from build123d import *

# Parameters (mm, degrees)
SKETCH1_W           = 39
SKETCH1_H           = 35
SKETCH1_R           = 1.912731322
BOSS_EXTRUDE1_DEPTH = 5
SKETCH2_R           = 2
BOSS_EXTRUDE2_DEPTH = 20
FILLET1_R           = 8


with BuildPart() as part:
    # Sketch1 → Boss-Extrude1 (new body)
    with BuildSketch(Plane.XY):
        Rectangle(SKETCH1_W, SKETCH1_H)
        with Locations((14.5, -12.5)):
            Circle(SKETCH1_R, mode=Mode.SUBTRACT)
        with Locations((14.5, 12.5)):
            Circle(SKETCH1_R, mode=Mode.SUBTRACT)
        with Locations((-14.5, -12.5)):
            Circle(SKETCH1_R, mode=Mode.SUBTRACT)
        with Locations((-14.5, 12.5)):
            Circle(SKETCH1_R, mode=Mode.SUBTRACT)
    extrude(amount=BOSS_EXTRUDE1_DEPTH)

    # Sketch2 → Boss-Extrude2 (add)
    with BuildSketch(Plane.XY.offset(5)):
        Circle(SKETCH2_R)
    extrude(amount=BOSS_EXTRUDE2_DEPTH)

    # Fillet1
    fillet1_edges = [part.edges().sort_by_distance(p)[0] for p in [
        (-2, 0, 5),
    ]]
    fillet(fillet1_edges, radius=FILLET1_R)


solid = part.part
Input: part model. Units: mm. Frame: model coordinates. A direction names the side the tool comes from. Coordinates: 2 decimals unless noted, no trailing zeros. Order: outer loops, then holes, each group sorted by start corner. A loop starts at its lowest first (then second) coordinate and runs counter-clockwise, first axis right, second up. Notation, with made-up numbers: M -5.5,57.25 L 8.5,57.25 A17 ccw 8.5,69.25 Z; hole C -26,-31.75 d10. An arc over 180 degrees is marked long. Write item = value, one per line. Start each with the question number.
(1) Line query: line 1 along Y through (x, z) = (-14.5, 2.3); line 2 along Z through (x, y) = (-14.5, -0.5); line 3 along X through (y, z) = (-0.5, 10.75). Output: solid intervals per line, ascending. Write a range as [from, to].
(2) Reachability of faces 1 (the flat face through (0, 0, 25)), 2 (the cylindrical face through (0, -2, 19)) from +Z, -Z, +X, -X, +Y, -Y: full face, straight path, thin tool, end or side. Return the list, or none.
(3) First-contact query: P1, Ø3, axis at x = -14.5, y = -12.5, coming from the +Z side; P2, Ø5, axis at x = -14.5, y = 12.5, coming from the +Z side; P3, Ø8, axis at y = 1, z = 14, coming from the -X side; P4, Ø3, axis at x = 2, z = 12, coming from the +Y side. Flat tips, straight axial feed; report the tip coordinate or a pass-through.
(4) Pull-direction query (Y, two-part tool) for faces 3 (the flat face through (0, -17.5, 2)), 4 (the cylindrical face through (-13.47, 14.11, 2.46)), 5 (the cylindrical face through (15.53, -10.89, 2.46)), 6 (the flat face through (-19.5, 0, 2)); classes: released by +Y, released by -Y, zero draft, split by the parting line, or undercut.
(5) Section A-A on x = -14.5. Output: boundary loops of the cut face in (y, z), and give its area (3 significant figures).
(6) Section D-D on z = 23.75. Output: boundary loops of the cut face in (x, y), and give its area (3 significant figures).
(7) Section C-C on x = 0. Output: boundary loops of the cut face in (y, z).
(8) Section B-B on y = 12.5. Output: boundary loops of the cut face in (x, z).
Result set:
q1.line_1 = [-17.5, -14.41], [-10.59, 10.59], [14.41, 17.5]
q1.line_2 = [0, 5]
q1.line_3 = [-2.27, 2.27]
q2.face_1 = +Z, +X, -X, +Y, -Y
q2.face_2 = +Z
q3.P1 = through
q3.P2 = 5
q3.P3 = -2.54
q3.P4 = 2.08
q4.face_3 = released by -Y
q4.face_4 = undercut
q4.face_5 = undercut
q4.face_6 = zero draft
q5.outline = M -17.5,0 L -14.41,0 L -14.41,5 L -17.5,5 Z; M -10.59,0 L 10.59,0 L 10.59,5 L -10.59,5 Z; M 14.41,0 L 17.5,0 L 17.5,5 L 14.41,5 Z
q5.area = 137 mm²
q6.outline = C 0,0 d4
q6.area = 12.6 mm²
q7.outline = M -17.5,0 L 17.5,0 L 17.5,5 L 10,5 A8 cw 2,13 L 2,25 L -2,25 L -2,13 A8 cw -10,5 L -17.5,5 Z
q8.outline = M -19.5,0 L -16.41,0 L -16.41,5 L -19.5,5 Z; M -12.59,0 L 12.59,0 L 12.59,5 L -12.59,5 Z; M 16.41,0 L 19.5,0 L 19.5,5 L 16.41,5 Z
